Job drawing, mm, ordinate dimensions from the low corner. One solid piece. A direction names the side the tool comes from. Give positions to 0.01 mm unless a question says otherwise; leave off trailing zeros. Order: outer loops, then holes, each group sorted by start corner. A loop starts at its lowest first (then second) coordinate and runs counter-clockwise, first axis right, second up.
1. Slice it at D-D on x = 26.25. List the corners of the cut face in (y, z).
2. Slice it at B-B on y = 13.5. List the corners of the cut face in (x, z).
3. Drop flat-ended pins along their axis: pin 1 Ø7.5 at (x, y) = (2, 10.5) entering from -Z; pin 2 Ø1.6 at (y, z) = (30, 9.5) entering from -X; pin 3 Ø13.5 at (x, z) = (19, 9) entering from -Y. Give the stop position or say it passes through.
4. Which spindle directions (+Z, -Z, +X, -X, +Y, -Y) get a long thin tool onto all of the face, cutting with end or side? Do the marked faces 4 and 5. Say none if no direction does.
5. Slice it at A-A on x = 15. List the corners of the cut face in (y, z), and give its area (3 significant figures).
6. Probe line 1 (X direction, y = 28, z = 21.75); line 2 (Z direction, x = 15, y = 29.8); line 3 (Y direction, x = 23, z = 26.25). List the from-to ranges inside material, lowest first.
7. Mould opens along Y. For the marked faces 1, 2 and 3 say: +Y half, -Y half, draft (parallel to the pull), parting line (faces both ways), or undercut.
8. Slice it at C-C on z = 22.5. List the corners of the cut face in (x, y), and give its area (4 significant figures).
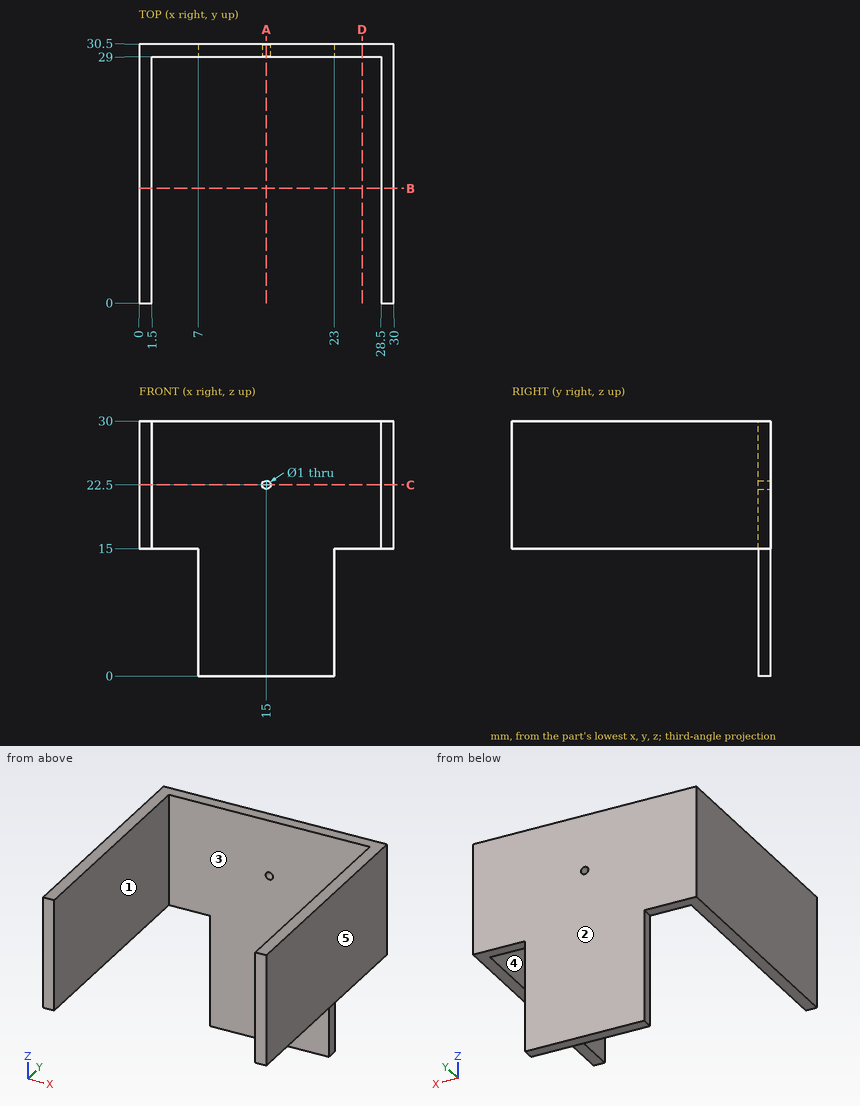
Data:
1. outline: (29, 15) - (30.5, 15) - (30.5, 30) - (29, 30) - close
2. outline: (0, 15) - (1.5, 15) - (1.5, 30) - (0, 30) - close; (28.5, 15) - (30, 15) - (30, 30) - (28.5, 30) - close
3. pin 1: stops at z = 15
3. pin 2: stops at x = 7
3. pin 3: stops at y = 29
4. face 4: +Z, -Z, -Y
4. face 5: +Z, -Z, +X, +Y, -Y
5. outline: (29, 0) - (30.5, 0) - (30.5, 22) - (29, 22) - close; (29, 23) - (30.5, 23) - (30.5, 30) - (29, 30) - close
5. area: 43.5 mm2
6. line 1: x = 0 to 1.5, 28.5 to 30
6. line 2: z = 0 to 22, 23 to 30
6. line 3: y = 29 to 30.5
7. face 1: draft
7. face 2: +Y half
7. face 3: -Y half
8. outline: (0, 0) - (1.5, 0) - (1.5, 29) - (14.5, 29) - (14.5, 30.5) - (0, 30.5) - close; (15.5, 29) - (28.5, 29) - (28.5, 0) - (30, 0) - (30, 30.5) - (15.5, 30.5) - close
8. area: 130.5 mm2
